Autodesk Inventor part; units mm, degrees
ref_plane "YZ Plane" through (0, 0, 0) normal (1, 0, 0) x (0, 1, 0)
ref_plane "XZ Plane" through (0, 0, 0) normal (0, 1, 0) x (-1, 0, 0)
ref_plane "XY Plane" through (0, 0, 0) normal (0, 0, 1) x (1, 0, 0)
sketch "Sketch1" plane through (0, 0, 0) normal (0, 1, 0) x (-1, 0, 0)
  line L0 (0, 0) -> (50, 0)
  line L1 (50, 0) -> (50, -5)
  line L2 (50, -5) -> (0, -5)
  line L3 (0, -5) -> (0, 0)
  line L4 (50, 0) -> (45, 0)
  line L5 (45, 0) -> (45, -50)
  line L6 (45, -50) -> (50, -50)
  line L7 (50, -50) -> (50, 0)
  point P0 (45, -5)
  dimension "d0" = 50
  dimension "d1" = 5
  dimension "d2" = 5
  dimension "d3" = 50
extrude "Extrusion1" add sketch "Sketch1" along normal blind 5
fillet "Fillet1" radius 2.5 8 edges at (-25, 5, 0) (-50, 5, -2.5) (-25, 0, 0) (-50, 0, -2.5) (-45, 0, -27.5) (-45, 5, -27.5) (-22.5, 5, -5) (-22.5, 0, -5)
properties part number "palanca"
Source: CAD feature listing. Evaluate the final solid. Frame: model axes, mm. A direction names the side the tool comes from. Round coordinates to 2 decimals unless told otherwise and drop trailing zeros. Loops run counter-clockwise (first coordinate to the right, second up) from the corner with the lowest first, then second, coordinate; pieces in that order, holes last. Notation, with made-up numbers: (-7, 77) -> (9, 77) arc R20 cw to (9, 94) -> close; hole circle Ø5 at (-36, -4). An arc over 180 degrees is marked (long way). Answer as a JSON object with one key per item and string values. Group by question number.
Q1. Access query for faces 1 (the cylindrical face through (-45.713, 0.752, -26.583)), 2 (the cylindrical face through (-23.417, 4.248, -4.287)), 3 (the cylindrical face through (-24.65, 0.752, -0.713)). Directions: +Z, -Z, +X, -X, +Y, -Y. A direction counts if a zero-diameter tool reaches every point of the face in a straight line with its end or side. Return the directions, or none.
Q2. Contact query for flat-ended pins moving along their axis: P1, Ø3, axis at y = 0.5, z = -39, coming from the -X side; P2, Ø2, axis at y = 4.5, z = -14, coming from the +X side. Output: stop coordinate, or through.
Q3. Section query D-D (y = 4.4). Output: boundary loops of the cut face in (x, z).
Q4. Ray query, line 1 (X direction, y = 2.4, z = -26.5); line 2 (Z direction, x = -23.5, y = 2.3); line 3 (Z direction, x = -44, y = 1.8). Return the intervals inside material, ascending. Write a range as from..to.
Q5. Section query C-C (y = 1.9). Output: boundary loops of the cut face in (x, z), plus the area to 3 significant figures.
Completed:
{
 "1": {"face 1": "-Z, +X, -Y", "face 2": "-Z, +X, +Y", "face 3": "+Z, +X, -X, -Y"},
 "2": {"P1": "x = -49.95", "P2": "x = -45.21"},
 "3": {"outline": "(-49.12, -50) -> (-45.88, -50) -> (-45.88, -4.12) -> (0, -4.12) -> (0, -0.88) -> (-49.12, -0.88) -> close"},
 "4": {"line 1": "-50..-45", "line 2": "-4.99..-0.01", "line 3": "-4.9..-0.1"},
 "5": {"outline": "(-49.93, -50) -> (-45.07, -50) -> (-45.07, -4.93) -> (0, -4.93) -> (0, -0.07) -> (-49.93, -0.07) -> close", "area": "461 mm²"}
}
